Geometry check sheet. Reference: the model listing, model coordinates, mm. Coordinates: 2 decimals unless noted, no trailing zeros. Loops run counter-clockwise (first coordinate to the right, second up) from the corner with the lowest first, then second, coordinate; pieces in that order, holes last.
from build123d import *

# Parameters (mm, degrees)
ESBO_O1_R                = 11
RESSALTO_EXTRUS_O1_DEPTH = 6
ESBO_O10_R               = 8
CORTE_EXTRUS_O4_DEPTH    = 5
CORTE_EXTRUS_O4_DRAFT    = -45
ESBO_O11_R               = 3
CORTE_EXTRUS_O5_DEPTH    = 17.340134638
FILETE4_R                = 1.5
FILETE5_R                = 1.5


with BuildPart() as part:
    # Esboço1 → Ressalto-extrusão1 (new body)
    with BuildSketch(Plane(origin=(0, 0, 0), x_dir=(1, 0, 0), z_dir=(0, 1, 0))):
        with Locations(Location((0, 0, 0), (0, 0, 270))):
            Circle(ESBO_O1_R)
    extrude(amount=RESSALTO_EXTRUS_O1_DEPTH)


with BuildPart() as corte_extrus_o4_tool:
    # Esboço10 → Corte-extrusão4 (with draft: the straight prism first)
    with BuildSketch(Plane.XZ):
        Circle(ESBO_O10_R)
    extrude(amount=-CORTE_EXTRUS_O4_DEPTH)
    # Corte-extrusão4: the draft: its side faces are tilted about the plane it starts from
    corte_extrus_o4_sides = [corte_extrus_o4_tool.faces().sort_by_distance(p)[0] for p in [
        (-8, 2.5, 0),
    ]]
    draft(corte_extrus_o4_sides, Plane.XZ, CORTE_EXTRUS_O4_DRAFT)


with BuildPart() as part_1:
    add(part.part)

    # Corte-extrusão4: cut by corte_extrus_o4_tool
    add(corte_extrus_o4_tool.part, mode=Mode.SUBTRACT)

    # Esboço11 → Corte-extrusão5 (cut, through all)
    with BuildSketch(Plane.XZ.offset(-5)):
        with Locations(Location((0, 0, 0), (0, 0, 270))):
            Circle(ESBO_O11_R)
    extrude(amount=-CORTE_EXTRUS_O5_DEPTH, mode=Mode.SUBTRACT)

    # Filete4
    filete4_edges = [part_1.edges().sort_by_distance(p)[0] for p in [
        (0, 0, -11),
    ]]
    fillet(filete4_edges, radius=FILETE4_R)

    # Filete5
    filete5_edges = [part_1.edges().sort_by_distance(p)[0] for p in [
        (0, 6, -11),
    ]]
    fillet(filete5_edges, radius=FILETE5_R)


solid = part_1.part
(1) Draft check along Z on faces 1 (the cylindrical face through (-10.74, 2.98, -2.38)), 2 (the conical face through (3.16, 4.687, 0.995)), 3 (the flat face through (-7, 0, -4.3)). Enter one of: +Z half, -Z half, draft (parallel to the pull), parting line (faces both ways), or undercut.
Findings:
face 1: parting line
face 2: undercut
face 3: draft
(2) Gauge pin test, flat ends, axial feed: pin 1 Ø10 at (x, z) = (-2.5, -8) entering from -Y; pin 2 Ø1.5 at (y, z) = (4.5, -3.5) entering from +X; pin 3 Ø2 at (y, z) = (3, -1.5) entering from -X; pin 4 Ø3 at (y, z) = (1.5, -4) entering from -X. Record the tip position at first contact, or that the pin passes through.
Findings:
pin 1: stops at y = 0
pin 2: stops at x = 10.65
pin 3: stops at x = -10.99
pin 4: stops at x = -10.71
(3) Sectioned sample at B-B on y = 2.6. Record the cut outline in (x, z).
Findings:
outline: circle Ø22 at (0, 0); hole circle Ø10.8 at (0, 0)
(4) Scan lines: L1, parallel to X at y = 0.35, z = -5.75; L2, parallel to X at y = 5.65, z = 0; L3, parallel to Z at x = 5.25, y = 1.9. Record each from-to range of solid material in increasing order.
Findings:
L1: x = -8.74 to -5.05, 5.05 to 8.74
L2: x = -10.46 to -3, 3 to 10.46
L3: z = -9.67 to -3.11, 3.11 to 9.67
(5) Sectioned sample at A-A on x = 0. Record the cut outline in (y, z), and give its area (3 significant figures).
Findings:
outline: (0, -9.5) arc R1.5 ccw to (1.5, -11) - (4.5, -11) arc R1.5 ccw to (6, -9.5) - (6, -3) - (5, -3) - (0, -8) - close; (0, 8) - (5, 3) - (6, 3) - (6, 9.5) arc R1.5 ccw to (4.5, 11) - (1.5, 11) arc R1.5 ccw to (0, 9.5) - close
area: 69.1 mm2
